```python
from build123d import *

# Parameters (mm, degrees)
EXTRUDE_1_DEPTH = 10


with BuildPart() as part:
    # 草图1 → 凸台-拉伸1 (new body)
    with BuildSketch(Plane.XY):
        with BuildLine():
            Line((66.531250095, 17), (73.031250095, 17))
            Line((73.031250095, 17), (73.031250095, 16))
            Line((73.031250095, 16), (75.831250095, 16))
            Line((75.831250095, 16), (75.831250095, 20))
            Line((75.831250095, 20), (60.031250095, 20))
            Line((60.031250095, 20), (44.231250095, 20))
            Line((44.231250095, 20), (44.231250095, 16))
            Line((44.231250095, 16), (47.031250095, 16))
            Line((47.031250095, 16), (47.031250095, 17))
            Line((47.031250095, 17), (53.531250095, 17))
            ThreePointArc((53.531250095, 17), (54.455129627, 16.382683432), (54.238356876, 15.292893219))
            Line((54.238356876, 15.292893219), (49.945463657, 11))
            Line((49.945463657, 11), (47.031250095, 11))
            Line((47.031250095, 11), (47.031250095, 9))
            Line((47.031250095, 9), (44.231250095, 9))
            Line((44.231250095, 9), (44.231250095, 7.2))
            ThreePointArc((44.231250095, 7.2), (40.031250095, 3), (35.831250095, 7.2))
            Line((35.831250095, 7.2), (35.831250095, 9))
            Line((35.831250095, 9), (33.031250095, 9))
            Line((33.031250095, 9), (33.031250095, 11))
            Line((33.031250095, 11), (30.117036532, 11))
            Line((30.117036532, 11), (25.824143314, 15.292893219))
            ThreePointArc((25.824143314, 15.292893219), (25.607370562, 16.382683432), (26.531250095, 17))
            Line((26.531250095, 17), (33.031250095, 17))
            Line((33.031250095, 17), (33.031250095, 16))
            Line((33.031250095, 16), (35.831250095, 16))
            Line((35.831250095, 16), (35.831250095, 20))
            Line((35.831250095, 20), (1.031250095, 20))
            ThreePointArc((1.031250095, 20), (0.324143314, 19.707106781), (0.031250095, 19))
            Line((0.031250095, 19), (0.031250095, 14.2))
            Line((0.031250095, 14.2), (4.031250095, 14.2))
            Line((4.031250095, 14.2), (4.031250095, 17))
            Line((4.031250095, 17), (11.031250095, 17))
            Line((11.031250095, 17), (11.031250095, 3))
            Line((11.031250095, 3), (4.031250095, 3))
            Line((4.031250095, 3), (4.031250095, 5.8))
            Line((4.031250095, 5.8), (0.031250095, 5.8))
            Line((0.031250095, 5.8), (0.031250095, 1))
            ThreePointArc((0.031250095, 1), (0.324143314, 0.292893219), (1.031250095, 0))
            Line((1.031250095, 0), (15.831250095, 0))
            Line((15.831250095, 0), (15.831250095, 4))
            Line((15.831250095, 4), (13.031250095, 4))
            Line((13.031250095, 4), (13.031250095, 11))
            Line((13.031250095, 11), (15.831250095, 11))
            Line((15.831250095, 11), (15.831250095, 12.8))
            ThreePointArc((15.831250095, 12.8), (20.031250095, 17), (24.231250095, 12.8))
            Line((24.231250095, 12.8), (24.231250095, 11))
            Line((24.231250095, 11), (27.031250095, 11))
            Line((27.031250095, 11), (27.031250095, 9))
            Line((27.031250095, 9), (29.945463657, 9))
            Line((29.945463657, 9), (34.238356876, 4.707106781))
            ThreePointArc((34.238356876, 4.707106781), (34.455129627, 3.617316568), (33.531250095, 3))
            Line((33.531250095, 3), (27.031250095, 3))
            Line((27.031250095, 3), (27.031250095, 4))
            Line((27.031250095, 4), (24.231250095, 4))
            Line((24.231250095, 4), (24.231250095, 0))
            Line((24.231250095, 0), (55.831250095, 0))
            Line((55.831250095, 0), (55.831250095, 4))
            Line((55.831250095, 4), (53.031250095, 4))
            Line((53.031250095, 4), (53.031250095, 3))
            Line((53.031250095, 3), (46.531250095, 3))
            ThreePointArc((46.531250095, 3), (45.607370562, 3.617316568), (45.824143314, 4.707106781))
            Line((45.824143314, 4.707106781), (50.117036532, 9))
            Line((50.117036532, 9), (53.031250095, 9))
            Line((53.031250095, 9), (53.031250095, 11))
            Line((53.031250095, 11), (55.831250095, 11))
            Line((55.831250095, 11), (55.831250095, 12.8))
            ThreePointArc((55.831250095, 12.8), (57.061401614, 15.769848481), (60.031250095, 17))
            ThreePointArc((60.031250095, 17), (63.001098576, 15.769848481), (64.231250095, 12.8))
            Line((64.231250095, 12.8), (64.231250095, 11))
            Line((64.231250095, 11), (67.031250095, 11))
            Line((67.031250095, 11), (67.031250095, 9))
            Line((67.031250095, 9), (69.945463657, 9))
            Line((69.945463657, 9), (74.238356876, 4.707106781))
            ThreePointArc((74.238356876, 4.707106781), (74.455129627, 3.617316568), (73.531250095, 3))
            Line((73.531250095, 3), (67.031250095, 3))
            Line((67.031250095, 3), (67.031250095, 4))
            Line((67.031250095, 4), (64.231250095, 4))
            Line((64.231250095, 4), (64.231250095, 0))
            Line((64.231250095, 0), (95.831250095, 0))
            Line((95.831250095, 0), (95.831250095, 4))
            Line((95.831250095, 4), (93.031250095, 4))
            Line((93.031250095, 4), (93.031250095, 3))
            Line((93.031250095, 3), (86.531250095, 3))
            ThreePointArc((86.531250095, 3), (85.607370562, 3.617316568), (85.824143314, 4.707106781))
            Line((85.824143314, 4.707106781), (90.117036532, 9))
            Line((90.117036532, 9), (93.031250095, 9))
            Line((93.031250095, 9), (93.031250095, 11))
            Line((93.031250095, 11), (95.831250095, 11))
            Line((95.831250095, 11), (95.831250095, 12.8))
            ThreePointArc((95.831250095, 12.8), (100.031250095, 17), (104.231250095, 12.8))
            Line((104.231250095, 12.8), (104.231250095, 11))
            Line((104.231250095, 11), (107.031250095, 11))
            Line((107.031250095, 11), (107.031250095, 4))
            Line((107.031250095, 4), (104.231250095, 4))
            Line((104.231250095, 4), (104.231250095, 0))
            Line((104.231250095, 0), (119.031250095, 0))
            ThreePointArc((119.031250095, 0), (119.738356876, 0.292893219), (120.031250095, 1))
            Line((120.031250095, 1), (120.031250095, 5.8))
            Line((120.031250095, 5.8), (116.031250095, 5.8))
            Line((116.031250095, 5.8), (116.031250095, 3))
            Line((116.031250095, 3), (109.031250095, 3))
            Line((109.031250095, 3), (109.031250095, 17))
            Line((109.031250095, 17), (116.031250095, 17))
            Line((116.031250095, 17), (116.031250095, 14.2))
            Line((116.031250095, 14.2), (120.031250095, 14.2))
            Line((120.031250095, 14.2), (120.031250095, 19))
            ThreePointArc((120.031250095, 19), (119.738356876, 19.707106781), (119.031250095, 20))
            Line((119.031250095, 20), (84.231250095, 20))
            Line((84.231250095, 20), (84.231250095, 16))
            Line((84.231250095, 16), (87.031250095, 16))
            Line((87.031250095, 16), (87.031250095, 17))
            Line((87.031250095, 17), (93.531250095, 17))
            ThreePointArc((93.531250095, 17), (94.455129627, 16.382683432), (94.238356876, 15.292893219))
            Line((94.238356876, 15.292893219), (89.945463657, 11))
            Line((89.945463657, 11), (87.031250095, 11))
            Line((87.031250095, 11), (87.031250095, 9))
            Line((87.031250095, 9), (84.231250095, 9))
            Line((84.231250095, 9), (84.231250095, 7.2))
            ThreePointArc((84.231250095, 7.2), (80.031250095, 3), (75.831250095, 7.2))
            Line((75.831250095, 7.2), (75.831250095, 9))
            Line((75.831250095, 9), (73.031250095, 9))
            Line((73.031250095, 9), (73.031250095, 11))
            Line((73.031250095, 11), (70.117036532, 11))
            Line((70.117036532, 11), (65.824143314, 15.292893219))
            ThreePointArc((65.824143314, 15.292893219), (65.607370562, 16.382683432), (66.531250095, 17))
        make_face()
    extrude(amount=EXTRUDE_1_DEPTH)


solid = part.part
```
Can you work these out from the model? Positions are in its coordinate system, mm. A direction names the side the tool comes from. Coordinates: 2 decimals unless noted, no trailing zeros. Loops run counter-clockwise (first coordinate to the right, second up) from the corner with the lowest first, then second, coordinate; pieces in that order, holes last.
Item 1: Suppose I cut it at A-A (y = 18). Please give me the cut outline in (x, z).
Answers below:
outline: (0.03, 0) - (35.83, 0) - (35.83, 10) - (0.03, 10) - close; (44.23, 0) - (75.83, 0) - (75.83, 10) - (44.23, 10) - close; (84.23, 0) - (120.03, 0) - (120.03, 10) - (84.23, 10) - close
Item 2: If we mould it in two halves opening along Y, with no side actions, what happens to faces 1 (the face through (44.231, 18, 5)), 2 (the face through (2, 14.2, 5)), 3 (the face through (102, 20, 5))? For each: released by +Y, released by -Y, zero draft, split by the parting line, or undercut.
Answers below:
face 1: zero draft
face 2: undercut
face 3: released by +Y
Item 3: Please list where these lines run through material, in increasing order: L1, parallel to X at y = 2, z = 5.25; L2, parallel to X at y = 8.5, z = 9.75; L3, parallel to X at y = 7.75, z = 7.75.
Answers below:
L1: x = 0.03 to 15.83, 24.23 to 55.83, 64.23 to 95.83, 104.23 to 120.03
L2: x = 11.03 to 13.03, 30.45 to 35.83, 44.23 to 49.62, 70.45 to 75.83, 84.23 to 89.62, 107.03 to 109.03
L3: x = 11.03 to 13.03, 31.2 to 35.83, 44.23 to 48.87, 71.2 to 75.83, 84.23 to 88.87, 107.03 to 109.03
Item 4: Which directions (+Z, -Z, +X, -X, +Y, -Y) give clear straight access to the entire face, cutting with the end or side of a thin tool? Please do faces 4 (the face through (30, 17, 5)), 5 (the face through (118, 5.8, 5)), 6 (the face through (84.231, 18, 5)), 7 (the face through (2, 5.8, 5)).
Answers below:
face 4: +Z, -Z
face 5: +Z, -Z, +X
face 6: +Z, -Z, +Y
face 7: +Z, -Z, -X
Item 5: I'm going to push flat-ended pins straight in: pin 1 (1 mm diameter, centred on y = 9, z = 5, fed in from -X); pin 2 (1 mm diameter, centred on x = 47.5, y = 12.5, fed in from -Z); pin 3 (3 mm diameter, centred on x = 51.5, z = 6.5, fed in from -Y); pin 4 (2 mm diameter, centred on y = 10, z = 5, fed in from +X). Where does each tip first touch, or does it pass through?
Answers below:
pin 1: stops at x = 11.03
pin 2: passes through
pin 3: stops at y = 0
pin 4: stops at x = 109.03
Item 6: Suppose I cut it at B-B (x = 59). Please give me the cut outline in (y, z).
Answers below:
outline: (16.87, 0) - (20, 0) - (20, 10) - (16.87, 10) - close
